For this review, take the finished solid that the model builds, in its own axes (mm). A direction names the side the tool comes from. Round coordinates to 2 decimals unless told otherwise and drop trailing zeros. Order: outer loops, then holes, each group sorted by start corner. A loop starts at its lowest first (then second) coordinate and runs counter-clockwise, first axis right, second up. Notation, with made-up numbers: M 33,59 L 41,59 A10 ccw 41,72 Z; hole C 43,-24 d8. An arc over 180 degrees is marked long. Use a Markdown table: item, result.
from build123d import *

# Parameters (mm, degrees)
SKETCH1_R           = 1.5
SKETCH1_W           = 3
SKETCH1_H           = 4
BOSS_EXTRUDE1_DEPTH = 3


with BuildPart() as part:
    # Sketch1 → Boss-Extrude1 (new body)
    with BuildSketch(Plane(origin=(0, 0, 0), x_dir=(1, 0, 0), z_dir=(0, 1, 0))):
        Polygon((16, 34), (40, 34), (40, 0), (0, 0), (0, 34), (3, 34), (3, 22), (16, 22), align=None)
        with Locations((19.3, 31.65)):
            Circle(SKETCH1_R, mode=Mode.SUBTRACT)
        with Locations((25.8, 4.64)):
            Circle(SKETCH1_R, mode=Mode.SUBTRACT)
        with Locations((4.5, 3.5)):
            Rectangle(SKETCH1_W, SKETCH1_H, mode=Mode.SUBTRACT)
        with Locations((35.5, 3.5)):
            Rectangle(SKETCH1_W, SKETCH1_H, mode=Mode.SUBTRACT)
    extrude(amount=BOSS_EXTRUDE1_DEPTH)


solid = part.part
Q1. Add section A-A (z = -31.65). Write out the cut boundary in (x, y).
Determined:
| item | result |
|---|---|
| outline | M 0,0 L 3,0 L 3,3 L 0,3 Z; M 16,0 L 17.8,0 L 17.8,3 L 16,3 Z; M 20.8,0 L 40,0 L 40,3 L 20.8,3 Z |
Q2. Wall thickness on line 1 along X through (y, z) = (1.3, -4.64); line 2 along X through (y, z) = (1.8, -31.65); line 3 along Z through (x, y) = (4.5, 0.9): over which ranges is each line inside the solid? List them lowest first. Write a range as [from, to].
Determined:
| item | result |
|---|---|
| line 1 | x = [0, 3], [6, 24.3], [27.3, 34], [37, 40] |
| line 2 | x = [0, 3], [16, 17.8], [20.8, 40] |
| line 3 | z = [-22, -5.5], [-1.5, 0] |
Q3. Draft analysis for pull direction Z (two halves, no side actions). For faces 4 (the flat face through (28, 1, -34)), 5 (the flat face through (35, 1, -5.5)), 6 (the flat face through (20, 3, -17)), state which applies: pulls with the +Z half, pulls with the -Z half, needs draft (parallel to the pull), parting line crosses it, or undercut.
Determined:
| item | result |
|---|---|
| face 4 | pulls with the -Z half |
| face 5 | undercut |
| face 6 | needs draft |
Q4. Machinability: for faces 1 (the flat face through (4, 1, -5.5)), 2 (the flat face through (40, 1, -17)), 3 (the flat face through (16, 1, -28)), which of the approach directions +Z, -Z, +X, -X, +Y, -Y give a long, thin tool a straight path to every point of the face, cutting with its end or side? Answer none if there is none.
Determined:
| item | result |
|---|---|
| face 1 | +Y, -Y |
| face 2 | +Z, -Z, +X, +Y, -Y |
| face 3 | -Z, +Y, -Y |
Q5. Add section B-B (x = 25.8). Write out the cut boundary in (y, z), then the cut area to 3 significant figures.
Determined:
| item | result |
|---|---|
| outline | M 0,-34 L 3,-34 L 3,-6.14 L 0,-6.14 Z; M 0,-3.14 L 3,-3.14 L 3,0 L 0,0 Z |
| area | 93.0 mm^2 |
Q6. Add section C-C (z = -4.64). Write out the cut boundary in (x, y).
Determined:
| item | result |
|---|---|
| outline | M 0,0 L 3,0 L 3,3 L 0,3 Z; M 6,0 L 24.3,0 L 24.3,3 L 6,3 Z; M 27.3,0 L 34,0 L 34,3 L 27.3,3 Z; M 37,0 L 40,0 L 40,3 L 37,3 Z |
Q7. Add section D-D (x = 36.5). Write out the cut boundary in (y, z), then the cut area to 3 significant figures.
Determined:
| item | result |
|---|---|
| outline | M 0,-34 L 3,-34 L 3,-5.5 L 0,-5.5 Z; M 0,-1.5 L 3,-1.5 L 3,0 L 0,0 Z |
| area | 90.0 mm^2 |
Q8. Clearance check with a flat-ended pin moving along its axis: pin 1 (1.5 mm diameter, centred on x = 13, y = 2, fed in from -Z). State where the tip first meets the part, or that it passes through.
Determined:
| item | result |
|---|---|
| pin 1 | stops at z = -22 |
